Model file for the job. Use its own axes, mm. A direction names the side the tool comes from. Give positions to 0.01 mm unless a question says otherwise; leave off trailing zeros. Return JSON: item names as keys, results as strings. Group by question number.
from build123d import *

# Parameters (mm, degrees)
F2_R     = 5.08
F3_SIZE2 = 0.510443
F3_SIZE  = 1.905


with BuildPart() as f1:
    # F0 (on Front) → F1 (revolve)
    with BuildSketch(Plane.XZ):
        with BuildLine():
            Line((0, 3.175), (0, 0))
            Line((0, 0), (63.5, 0))
            ThreePointArc((63.5, 0), (60.710192, 6.735192), (53.975, 9.525))
            Line((53.975, 9.525), (20.805025, 9.525))
            ThreePointArc((20.805025, 9.525), (14.711283, 7.812062), (10.402513, 3.175))
            Line((10.402513, 3.175), (0, 3.175))
        make_face()
    revolve(axis=Axis((31.75, 0, 0), (-1, 0, 0)))

    # F2
    f2_edges = [f1.edges().sort_by_distance(p)[0] for p in [
        (10.402513, 0, -3.175),
    ]]
    fillet(f2_edges, radius=F2_R)

    # F3
    f3_edges = [f1.edges().sort_by_distance(p)[0] for p in [
        (0, 0, -3.175),
    ]]
    chamfer(f3_edges, length=F3_SIZE, length2=F3_SIZE2)


solid = f1.part
(1) Drop flat-ended pins along their axis: pin 1 Ø1.5 at (y, z) = (-7, -0.5) entering from +X; pin 2 Ø1.5 at (x, y) = (31, 7) entering from +Z; pin 3 Ø1.5 at (x, y) = (57, 1) entering from +Z. Give the stop position or say it passes through.
(2) Drill centre lines: L1, parallel to Y at x = 27, z = 0.25; L2, parallel to Z at x = 10, y = 1.25; L3, parallel to Y at x = 35, z = 4. Where is each one in solid material? Low to high.
(3) 3-axis set-ups, long thin cutter, end or side, ignore diameter. For faces 1 (the face through (4.74, -3.1, -0.69)), 2 (the face through (37.158, -5.796, -7.559)): which of +Z, -Z, +X, -X, +Y, -Y reach the whole face in a straight line?
Result set:
{
 "1": {"pin 1": "stops at x = 61.15", "pin 2": "stops at z = 7.19", "pin 3": "stops at z = 9.21"},
 "2": {"L1": "y = -9.52 to 9.52", "L2": "z = -3.53 to 3.53", "L3": "y = -8.64 to 8.64"},
 "3": {"face 1": "-X", "face 2": "+X, -X"}
}
